Here's how the part is built. I have some questions about the finished solid (model axes, mm). A direction names the side the tool comes from. Round coordinates to 2 decimals unless told otherwise and drop trailing zeros. Loops run counter-clockwise (first coordinate to the right, second up) from the corner with the lowest first, then second, coordinate; pieces in that order, holes last. Notation, with made-up numbers: M 0,-16 L 27,-16 A29 cw 27,5 Z; hole C 39.25,66.5 d6. An arc over 180 degrees is marked long. Write each question's results on one line, items separated by ' | '. Start each with the question number.
```python
from build123d import *

# Parameters (mm, degrees)
SKETCH1_R           = 1.524000008
SKETCH1_R_2         = 1.523999992
BOSS_EXTRUDE1_DEPTH = 1.575


with BuildPart() as part:
    # Sketch1 → Boss-Extrude1 (new body)
    with BuildSketch(Plane(origin=(0, 0, 0), x_dir=(1, 0, 0), z_dir=(0, 1, 0))):
        with BuildLine():
            Line((44.351293307, -40.014412246), (36.727293315, -40.014412246))
            Line((36.727293315, -40.014412246), (36.727293315, -46.615946892))
            Line((36.727293315, -46.615946892), (30.377293307, -46.615946892))
            Line((30.377293307, -46.615946892), (-29.674706693, -46.615946892))
            Line((-29.674706693, -46.615946892), (-36.024706701, -46.615946892))
            Line((-36.024706701, -46.615946892), (-36.024706701, -40.014412246))
            Line((-36.024706701, -40.014412246), (-43.648706693, -40.014412246))
            Line((-43.648706693, -40.014412246), (-43.648706693, -30.885946892))
            ThreePointArc((-43.648706693, -30.885946892), (-43.276732305, -29.98792128), (-42.378706693, -29.615946892))
            Line((-42.378706693, -29.615946892), (-38.043706693, -29.615946892))
            ThreePointArc((-38.043706693, -29.615946892), (-37.145681081, -29.243972504), (-36.773706693, -28.345946892))
            Line((-36.773706693, -28.345946892), (-36.773706693, -10.370428445))
            Line((-36.773706693, -10.370428445), (-12.148706693, -10.370428445))
            Line((-12.148706693, -10.370428445), (-12.148706693, -17.871301308))
            Line((-12.148706693, -17.871301308), (-12.148706693, -34.615947016))
            Line((-12.148706693, -34.615947016), (12.851293307, -34.615947016))
            Line((12.851293307, -34.615947016), (12.851293307, -17.871301308))
            Line((12.851293307, -17.871301308), (12.851293307, -10.370428445))
            Line((12.851293307, -10.370428445), (37.476293307, -10.370428445))
            Line((37.476293307, -10.370428445), (37.476293307, -28.345946892))
            ThreePointArc((37.476293307, -28.345946892), (37.848267695, -29.243972504), (38.746293307, -29.615946892))
            Line((38.746293307, -29.615946892), (42.351293307, -29.615946892))
            ThreePointArc((42.351293307, -29.615946892), (43.76550687, -30.20173333), (44.351293307, -31.615946892))
            Line((44.351293307, -31.615946892), (44.351293307, -40.014412246))
        make_face()
        with Locations(Location((-36.024706701, -35.965946892, 0), (0, 0, 270))):
            Circle(SKETCH1_R, mode=Mode.SUBTRACT)
        with Locations(Location((36.727293315, -35.947946892, 0), (0, 0, 270))):
            Circle(SKETCH1_R_2, mode=Mode.SUBTRACT)
    extrude(amount=BOSS_EXTRUDE1_DEPTH)


solid = part.part
```
Item 1: If we mould it in two halves opening along X, with no side actions, what happens to faces 5 (the face through (-36.025, 1, 43)), 6 (the face through (1, 1, 46.616)), 7 (the face through (0, 1, 34.616))? For each: released by +X, released by -X, zero draft, split by the parting line, or undercut.
Item 2: If we section it at B-B on y = 1.15: Please give me the cut outline in (x, z).
Item 3: If we section it at C-C on z = 43: Please give me the cut outline in (x, y) (3 decimals), and give its area (3 significant figures).
Item 4: I need wall thicknesses on L1, parallel to X at y = 0.1, z = 15; L2, parallel to X at y = 0.6, z = 32; L3, parallel to Z at x = -37, y = 1.3. Which ranges of each line are inside material? Lowest first, please.
Item 5: I'm going to push flat-ended pins straight in: pin 1 (5 mm diameter, centred on x = 36.73, z = 35.95, fed in from -Y); pin 2 (0.5 mm diameter, centred on y = 1, z = 23, fed in from +X); pin 3 (0.5 mm diameter, centred on x = 41.5, y = 1, fed in from +Z); pin 4 (0.5 mm diameter, centred on y = 1, z = 26.5, fed in from -X). Where does each tip first touch, or does it pass through?
Item 6: Which directions (+Z, -Z, +X, -X, +Y, -Y) give clear straight access to the entire face, cutting with the end or side of a thin tool? Please do faces 1 (the face through (-40, 1, 29.616)), 2 (the face through (-12.149, 1, 22)), 3 (the face through (37.476, 1, 19)), 4 (the face through (41, 1, 40.014)).
Item 7: If we section it at A-A on z = 19: Please give me the cut outline in (x, y) (3 decimals), and give its area (3 significant figures).
Item 8: If we section it at D-D on x = 5.5: Please give me the cut outline in (y, z) (3 decimals), and give its area (3 significant figures).
Numbers:
1) face 5: released by -X | face 6: zero draft | face 7: undercut
2) outline: M -43.65,30.89 A1.27 ccw -42.38,29.62 L -38.04,29.62 A1.27 cw -36.77,28.35 L -36.77,10.37 L -12.15,10.37 L -12.15,34.62 L 12.85,34.62 L 12.85,10.37 L 37.48,10.37 L 37.48,28.35 A1.27 cw 38.75,29.62 L 42.35,29.62 A2 ccw 44.35,31.62 L 44.35,40.01 L 36.73,40.01 L 36.73,46.62 L -36.02,46.62 L -36.02,40.01 L -43.65,40.01 Z; hole C -36.02,35.97 d3.05; hole C 36.73,35.95 d3.05
3) outline: M -36.025,0 L 36.727,0 L 36.727,1.575 L -36.025,1.575 Z | area: 115 mm²
4) L1: -36.77 to -12.15, 12.85 to 37.48 | L2: -43.65 to -12.15, 12.85 to 44.35 | L3: 29.07 to 34.79, 37.14 to 40.01
5) pin 1: y = 0 | pin 2: x = 37.48 | pin 3: z = 40.01 | pin 4: x = -36.77
6) face 1: -Z, -X, +Y, -Y | face 2: -Z, +Y, -Y | face 3: -Z, +X, +Y, -Y | face 4: +Z, +X, +Y, -Y
7) outline: M -36.774,0 L -12.149,0 L -12.149,1.575 L -36.774,1.575 Z; M 12.851,0 L 37.476,0 L 37.476,1.575 L 12.851,1.575 Z | area: 77.6 mm²
8) outline: M 0,34.616 L 1.575,34.616 L 1.575,46.616 L 0,46.616 Z | area: 18.9 mm²
